Work out the finished part from the listing and answer in its coordinate system (mm). Face numbers are marked on the shaded views. A direction names the side the tool comes from. Give positions to 0.01 mm unless a question says otherwise; leave off trailing zeros. Loops run counter-clockwise (first coordinate to the right, second up) from the corner with the lowest first, then second, coordinate; pieces in that order, holes last. Notation, with made-up numbers: (88, -35.5) - (104, -35.5) arc R21 cw to (104, -3.5) - close; hole circle Ø8 at (1.25, 35). An arc over 180 degrees is marked (long way). One line per question, with ' | ' between items.
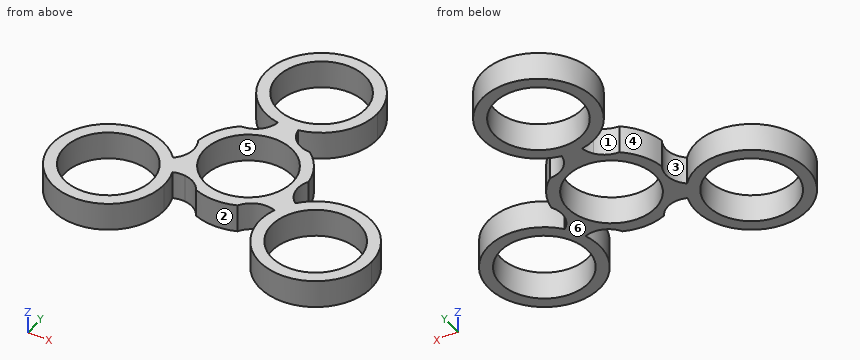
from build123d import *

# Parameters (mm, degrees)
F0_R     = 11
F1_DEPTH = 7


with BuildPart() as f1:
    # F0 (on Top) → F1 (new body)
    with BuildSketch(Plane.XY):
        with BuildLine():
            Line((14.05794, -8.116355), (15.328937, -5.914923))
            ThreePointArc((15.328937, -5.914923), (13.856406, -8), (12.786942, -10.317787))
            Line((12.786942, -10.317787), (14.05794, -8.116355))
        make_face()
        with BuildLine():
            ThreePointArc((39.980762, -15), (30.821963, -1.863685), (15.328937, -5.914923))
            Line((15.328937, -5.914923), (14.05794, -8.116355))
            Line((14.05794, -8.116355), (12.786942, -10.317787))
            ThreePointArc((12.786942, -10.317787), (23.605207, -28.796983), (39.980762, -15))
        make_face()
        with Locations((25.980762, -15)):
            Circle(F0_R, mode=Mode.SUBTRACT)
        with BuildLine():
            ThreePointArc((2.541994, 16.23271), (0, 16), (-2.541994, 16.23271))
            ThreePointArc((-2.541994, 16.23271), (-2.9479, 14.800569), (-3.683807, 13.506649))
            ThreePointArc((-3.683807, 13.506649), (-5.874203, 11.662049), (-8.660254, 11))
            ThreePointArc((-8.660254, 11), (-12.124356, 7), (-13.856406, 2))
            ThreePointArc((-13.856406, 2), (-13.131153, -2.22937), (-15.328937, -5.914923))
            ThreePointArc((-15.328937, -5.914923), (-13.856406, -8), (-12.786942, -10.317787))
            ThreePointArc((-12.786942, -10.317787), (-11.343719, -9.953241), (-9.855198, -9.943595))
            ThreePointArc((-9.855198, -9.943595), (-7.162529, -10.918233), (-5.196152, -13))
            ThreePointArc((-5.196152, -13), (0, -14), (5.196152, -13))
            ThreePointArc((5.196152, -13), (8.496267, -10.257227), (12.786942, -10.317787))
            ThreePointArc((12.786942, -10.317787), (13.856406, -8), (15.328937, -5.914923))
            ThreePointArc((15.328937, -5.914923), (14.291619, -4.847328), (13.539005, -3.563054))
            ThreePointArc((13.539005, -3.563054), (13.036732, -0.743815), (13.856406, 2))
            ThreePointArc((13.856406, 2), (12.124356, 7), (8.660254, 11))
            ThreePointArc((8.660254, 11), (4.634886, 12.486597), (2.541994, 16.23271))
        make_face()
        Circle(F0_R, mode=Mode.SUBTRACT)
        with BuildLine():
            ThreePointArc((-12.786942, -10.317787), (-13.856406, -8), (-15.328937, -5.914923))
            Line((-15.328937, -5.914923), (-14.05794, -8.116355))
            Line((-14.05794, -8.116355), (-12.786942, -10.317787))
        make_face()
        with BuildLine():
            Line((-14.05794, -8.116355), (-15.328937, -5.914923))
            ThreePointArc((-15.328937, -5.914923), (-39.117077, -19.8412), (-11.980762, -15))
            ThreePointArc((-11.980762, -15), (-12.183779, -12.624445), (-12.786942, -10.317787))
            Line((-12.786942, -10.317787), (-14.05794, -8.116355))
        make_face()
        with Locations((-25.980762, -15)):
            Circle(F0_R, mode=Mode.SUBTRACT)
        with BuildLine():
            ThreePointArc((2.541994, 16.23271), (10.76076, 21.044218), (14, 30))
            ThreePointArc((14, 30), (-8.955782, 40.76076), (-2.541994, 16.23271))
            Line((-2.541994, 16.23271), (0, 16.23271))
            Line((0, 16.23271), (2.541994, 16.23271))
        make_face()
        with Locations((0, 30)):
            Circle(F0_R, mode=Mode.SUBTRACT)
        with BuildLine():
            Line((0, 16.23271), (-2.541994, 16.23271))
            ThreePointArc((-2.541994, 16.23271), (0, 16), (2.541994, 16.23271))
            Line((2.541994, 16.23271), (0, 16.23271))
        make_face()
    extrude(amount=F1_DEPTH)


solid = f1.part
1. Find section C-C on y = -23.5. Write down the section's boundary in (x, z), then the cut area to 3 significant figures.
Evaluation:
outline: (-37.11, 0) - (-32.96, 0) - (-32.96, 7) - (-37.11, 7) - close; (-19, 0) - (-14.86, 0) - (-14.86, 7) - (-19, 7) - close; (14.86, 0) - (19, 0) - (19, 7) - (14.86, 7) - close; (32.96, 0) - (37.11, 0) - (37.11, 7) - (32.96, 7) - close | area: 116 mm2
2. Determine the mould class of the marked faces 4, 5 and 6 for opening direction X: +X half, -X half, draft (parallel to the pull), parting line (faces both ways), or undercut.
Evaluation:
face 4: -X half | face 5: undercut | face 6: draft
3. Find section D-D on y = 39.5. Write down the section's boundary in (x, z).
Evaluation:
outline: (-10.28, 0) - (-5.55, 0) - (-5.55, 7) - (-10.28, 7) - close; (5.55, 0) - (10.28, 0) - (10.28, 7) - (5.55, 7) - close
4. Flat-ended cylindrical pins translate along their axes: pin 1 (17.5 mm diameter, centred on x = 0, y = 30, fed in from +Z); pin 2 (1 mm diameter, centred on x = 18.5, z = 3, fed in from -Y); pin 3 (1 mm diameter, centred on y = -3.5, z = 6, fed in from -X). Find the tip coordinate at first contact, or state that the pin passes through.
Evaluation:
pin 1: through | pin 2: y = -27.14 | pin 3: x = -34.64
5. Consider L1, parallel to Y at x = 10, z = 1.75; L2, parallel to Y at x = -8, z = 6.5; L3, parallel to X at y = -20.5, z = 1.75. Determine where each line is inside the solid, lowest interval first.
Evaluation:
L1: -9.93 to -4.58, 4.58 to 9.8, 20.2 to 25.42, 34.58 to 39.8 | L2: -10.46 to -7.55, 7.55 to 11.04, 18.51 to 22.45, 37.55 to 41.49 | L3: -38.86 to -35.51, -16.45 to -13.11, 13.11 to 16.45, 35.51 to 38.86
6. Which of the six approach directions +Z, -Z, +X, -X, +Y, -Y give full straight-line access (tool end or side, diameter ignored) to the marked faces 1, 2 and 3?
Evaluation:
face 1: +Z, -Z, -X | face 2: +Z, -Z, -Y | face 3: +Z, -Z
7. Find section A-A on x = 0. Write down the section's boundary in (y, z).
Evaluation:
outline: (-14, 0) - (-11, 0) - (-11, 7) - (-14, 7) - close; (11, 0) - (19, 0) - (19, 7) - (11, 7) - close; (41, 0) - (44, 0) - (44, 7) - (41, 7) - close
8. Find section B-B on z = 5.5. Write down the section's boundary in (x, y), then the cut area to 3 significant figures.
Evaluation:
outline: (-15.33, -5.91) arc R14 ccw (long way) to (-11.98, -15) arc R14 ccw to (-12.79, -10.32) arc R6.19 cw to (-9.86, -9.94) arc R6.19 cw to (-5.2, -13) arc R14 ccw to (5.2, -13) arc R6.19 cw to (12.79, -10.32) arc R14 ccw (long way) to (15.33, -5.91) arc R6.19 cw to (13.54, -3.56) arc R6.19 cw to (13.86, 2) arc R14 ccw to (8.66, 11) arc R6.19 cw to (2.54, 16.23) arc R14 ccw to (14, 30) arc R14 ccw (long way) to (-2.54, 16.23) arc R6.19 cw to (-3.68, 13.51) arc R6.19 cw to (-8.66, 11) arc R14 ccw to (-13.86, 2) arc R6.19 cw to start; hole circle Ø22 at (-25.98, -15); hole circle Ø22 at (0, 0); hole circle Ø22 at (0, 30); hole circle Ø22 at (25.98, -15) | area: 960 mm2
